Can you work these out from the model? Positions are in its coordinate system, mm. A direction names the side the tool comes from. Coordinates: 2 decimals unless noted, no trailing zeros. Write each loop counter-clockwise with the first axis right and the second up, starting at its lowest first coordinate (ties: lowest second). Pieces come first, ordered by that corner, then holes. Notation, with made-up numbers: (-14.5, 52) - (18.5, 52) arc R27 ccw to (18.5, 87) - close; hole circle Ø1 at (5.5, 72). An arc over 180 degrees is marked (long way). Write each question's results on one line, items separated by ' | '. Start each with the question number.
```python
from build123d import *

# Parameters (mm, degrees)
F0_W     = 76.2
F0_H     = 76.2
F0_R     = 5.08
F0_R_2   = 19.05
F1_DEPTH = 1.8796
F2_R     = 5.08
F5_W     = 45.474999
F5_H     = 38.948495
F6_DEPTH = 47.498


with BuildPart() as f1:
    # F0 (on Top) → F1 (new body)
    with BuildSketch(Plane.XY):
        Rectangle(F0_W, F0_H)
        with Locations((-27.94, -27.94)):
            Circle(F0_R, mode=Mode.SUBTRACT)
        with Locations((27.94, -27.94)):
            Circle(F0_R, mode=Mode.SUBTRACT)
        with Locations((-27.94, 27.94)):
            Circle(F0_R, mode=Mode.SUBTRACT)
        Circle(F0_R_2, mode=Mode.SUBTRACT)
        with Locations((27.94, 27.94)):
            Circle(F0_R, mode=Mode.SUBTRACT)
    extrude(amount=F1_DEPTH)

    # F2
    f2_edges = [f1.edges().sort_by_distance(p)[0] for p in [
        (-38.1, -38.1, 0.9398),
        (38.1, -38.1, 0.9398),
        (38.1, 38.1, 0.9398),
        (-38.1, 38.1, 0.9398),
    ]]
    fillet(f2_edges, radius=F2_R)

    # F5 (on face) → F6 (join)
    with BuildSketch(Plane.XY.offset(1.8796)):
        with Locations((0.315798, -2.315857)):
            Rectangle(F5_W, F5_H)
    extrude(amount=F6_DEPTH)


solid = f1.part
```
Q1. Thinking about a two-plate mould opening in X: for faces 4 (the face through (-9, 17, 0)), 5 (the face through (-36.651, 36.572, 0.953)), 6 (the face through (32.785, 29.466, 0.927)), 7 (the face through (38.1, 0, 1)), which applies, pulls with the +X half, pulls with the -X half, needs draft (parallel to the pull), parting line crosses it, or undercut?
Q2. I need wall thicknesses on line 1 along Y through (x, z) = (-27.94, 1); line 2 along Y through (x, z) = (-27, 1); line 3 along Y through (x, z) = (-6, 45). Which ranges of each line are inside material? Lowest first, please. Write a range as from..to.
Q3. If we section it at A-A (x = 0): Please give me the cut outline in (y, z), then the cut area to 3 significant figures.
Q4. For faces 1 (the face through (-22.422, -3, 25)), 2 (the face through (0, -21.79, 25)), 3 (the face through (0, 17.158, 25)), which set-ups out of +Z, -Z, +X, -X, +Y, -Y let a thin tool reach every point of the face, with its end or its side?
Q5. I'm going to push flat-ended pins straight in: pin 1 Ø22.5 at (x, z) = (4, 24) entering from +Y; pin 2 Ø10 at (y, z) = (-0.5, 23) entering from +X; pin 3 Ø19.5 at (y, z) = (-8.5, 31) entering from -X; pin 4 Ø9 at (x, y) = (27.94, -27.94) entering from +Z. Where does each tip first touch, or does it pass through?
Q6. If we section it at D-D (z = 15.5): Please give me the cut outline in (x, y).
Q7. If we section it at B-B (x = 27.94): Please give me the cut outline in (y, z).
Answer list:
1) face 4: needs draft | face 5: pulls with the -X half | face 6: undercut | face 7: pulls with the +X half
2) line 1: y = -38.1..-33.02, -22.86..22.86, 33.02..38.1 | line 2: y = -38.1..-32.93, -22.95..22.95, 32.93..38.1 | line 3: y = -21.79..17.16
3) outline: (-38.1, 0) - (-19.05, 0) - (-19.05, 1.88) - (17.16, 1.88) - (17.16, 49.38) - (-21.79, 49.38) - (-21.79, 1.88) - (-38.1, 1.88) - close; (19.05, 0) - (38.1, 0) - (38.1, 1.88) - (19.05, 1.88) - close | area: 1,920 mm2
4) face 1: +Z, -X, +Y, -Y | face 2: +Z, +X, -X, -Y | face 3: +Z, +X, -X, +Y
5) pin 1: stops at y = 17.16 | pin 2: stops at x = 23.05 | pin 3: stops at x = -22.42 | pin 4: passes through
6) outline: (-22.42, -21.79) - (23.05, -21.79) - (23.05, 17.16) - (-22.42, 17.16) - close
7) outline: (-38.1, 0) - (-33.02, 0) - (-33.02, 1.88) - (-38.1, 1.88) - close; (-22.86, 0) - (22.86, 0) - (22.86, 1.88) - (-22.86, 1.88) - close; (33.02, 0) - (38.1, 0) - (38.1, 1.88) - (33.02, 1.88) - close
